Read the model definition and answer for the solid it produces. Units are mm, in the model's axes. Face numbers are marked on the shaded views. A direction names the side the tool comes from. Round coordinates to 2 decimals unless told otherwise and drop trailing zeros. Write each loop counter-clockwise with the first axis right and the second up, starting at its lowest first coordinate (ties: lowest second). Pieces come first, ordered by that corner, then holes. Notation, with made-up numbers: (-32.5, 11.25) - (-8.5, 11.25) arc R7 cw to (-8.5, 18.25) - close; hole circle Ø8 at (-7, 33.5). An arc over 180 degrees is marked (long way). Answer as CSV lines item,"result". Start each with the question number.
1) Which of the six approach directions +Z, -Z, +X, -X, +Y, -Y give full straight-line access (tool end or side, diameter ignored) to the marked faces 1 and 2?
2) Find section A-A on y = 2. Determine the outline of the cut face in (x, z), then the cut area to 3 significant figures.
3) Consider line 1 along Y through (x, z) = (14, 21). Determine where the line is inside the solid, lowest interval first.
4) Find section C-C on z = 22. Determine the outline of the cut face in (x, y).
5) For a pull along X with two mould halves and no side action, classify the marked faces 3, 4 and 5 as +X half, -X half, draft (parallel to the pull), parting line (faces both ways), or undercut.
from build123d import *

# Parameters (mm, degrees)
F1_START = 3
F1_DEPTH = 51


with BuildPart() as f1:
    # F0 (on Top) → F1 (new body)
    with BuildSketch(Plane.XY.offset(F1_START)):
        Polygon((0, 0), (0, 70), (69.8, 70), (69.8, 73), (-3, 73), (-3, -3), (73, -3), (73, 73), (70, 73), (70, 70), (70, 0), align=None)
    extrude(amount=F1_DEPTH)


solid = f1.part
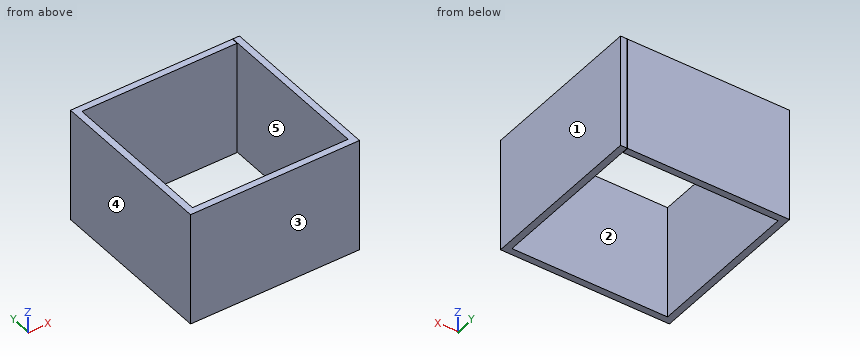
Check values:
1,face 1,"+Z, -Z, +X, +Y, -Y"
1,face 2,"+Z, -Z"
2,outline,"(-3, 3) - (0, 3) - (0, 54) - (-3, 54) - close; (70, 3) - (73, 3) - (73, 54) - (70, 54) - close"
2,area,"306 mm^2"
3,line 1,"y = -3 to 0, 70 to 73"
4,outline,"(-3, -3) - (73, -3) - (73, 73) - (70, 73) - (70, 0) - (0, 0) - (0, 70) - (69.8, 70) - (69.8, 73) - (-3, 73) - close"
5,face 3,"draft"
5,face 4,"-X half"
5,face 5,"undercut"
